```python
from build123d import *

# Parameters (mm, degrees)
F1_DEPTH = 82.55
F2_W     = 25.4
F2_H     = 69.85
F3_DEPTH = 82.55
F4_R     = 20.6375
F4_R_2   = 21.729164
F5_DEPTH = 25.4
F7_DEPTH = 25.4
F8_R     = 23.8125
F9_DEPTH = 25.4


with BuildPart() as f1:
    # F0 (on Front) → F1 (new body)
    with BuildSketch(Plane.XZ):
        Polygon((0, 57.15), (0, 0), (190.5, 0), (190.5, 12.7), (25.4, 12.7), (25.4, 57.15), align=None)
    extrude(amount=F1_DEPTH)

    # F2 (on face) → F3 (join)
    with BuildSketch(Plane.XZ.offset(82.55)):
        with Locations((12.7, 92.075)):
            Rectangle(F2_W, F2_H)
    extrude(amount=-F3_DEPTH)

    # F4 (on face) → F5 (cut)
    with BuildSketch(Plane.XY.offset(12.7)):
        with Locations((76.2, -41.275)):
            Circle(F4_R)
        with Locations((152.4, -41.275)):
            Circle(F4_R_2)
    extrude(amount=-F5_DEPTH, mode=Mode.SUBTRACT)

    # F6 (on face) → F7 (cut)
    with BuildSketch(Plane.YZ.offset(25.4)):
        with BuildLine():
            ThreePointArc((-82.55, 69.85), (-41.275, 111.125), (0, 69.85))
            Line((0, 69.85), (0, 127))
            Line((0, 127), (-82.55, 127))
            Line((-82.55, 127), (-82.55, 69.85))
        make_face()
    extrude(amount=-F7_DEPTH, mode=Mode.SUBTRACT)

    # F8 (on face) → F9 (cut)
    with BuildSketch(Plane.YZ.offset(25.4)):
        with Locations((-41.145787, 70.089974)):
            Circle(F8_R)
    extrude(amount=-F9_DEPTH, mode=Mode.SUBTRACT)


solid = f1.part
```
Geometry check sheet. Reference: the model listing, model coordinates, mm. A direction names the side the tool comes from. Give positions to 0.01 mm unless a question says otherwise; leave off trailing zeros. Order: outer loops, then holes, each group sorted by start corner. A loop starts at its lowest first (then second) coordinate and runs counter-clockwise, first axis right, second up. Notation, with made-up numbers: (-37, 61) - (20, 61) arc R27 ccw to (20, 78) - close; hole circle Ø6 at (27, 14.25). An arc over 180 degrees is marked (long way). Answer in a Markdown table with one row per item. Add a question column.
Q1. Cross-section at B-B, the plane y = -24. Enter the section's corners in (x, z), then the cut area to 3 significant figures.
Q2. Gauge pin test, flat ends, axial feed: pin 1 (8 mm diameter, centred on y = -31.5, z = 89.5, fed in from +X); pin 2 (12 mm diameter, centred on x = 52, y = -66.5, fed in from +Z). Record the tip position at first contact, or that the pin passes through.
Q3. Tool access check on faces 1 (the cylindrical face through (149.57, -19.73, 6.44)), 2 (the flat face through (109, -41, 12.7)). Record the directions out of +Z, -Z, +X, -X, +Y, -Y that give a thin tool (end or side, any length) a straight path to the whole face; none if there is none.
Q4. Cross-section at C-C, the plane z = 73.5. Enter the section's corners in (x, y).
Q5. Material ranges on probe 1 along Y at (x, z) = (76.2, 3.25); probe 2 along X at (y, z) = (-55, 8); probe 3 along Z at (x, y) = (116, -42), recorded low to high. Write a range as from..to.
Q6. Mould release check, pull along Y, two halves, no side actions. Record for faces 3 (the cylindrical face through (12.878, -42.183, 111.115)), 4 (the flat face through (190.5, -41, 6)), 5 (the cylindrical face through (95.884, -35.076, 6.439)), 6 (the flat face through (60, 0, 12)): pulls with the +Y half, pulls with the -Y half, needs draft (parallel to the pull), parting line crosses it, or undercut.
Q7. Cross-section at A-A, the plane x = 76.2. Enter the section's corners in (y, z), then the cut area to 3 significant figures.
Check values:
| question | item | result |
|---|---|---|
| 1 | outline | (0, 0) - (64.91, 0) - (64.91, 12.7) - (25.4, 12.7) - (25.4, 53.57) - (0, 53.57) - close; (0, 86.61) - (25.4, 86.61) - (25.4, 107.34) - (0, 107.34) - close; (87.49, 0) - (139.22, 0) - (139.22, 12.7) - (87.49, 12.7) - close; (165.58, 0) - (190.5, 0) - (190.5, 12.7) - (165.58, 12.7) - close |
| 1 | area | 3,360 mm^2 |
| 2 | pin 1 | stops at x = 25.4 |
| 2 | pin 2 | stops at z = 12.7 |
| 3 | face 1 | +Z, -Z |
| 3 | face 2 | +Z, +X, +Y, -Y |
| 4 | outline | (0, -82.39) - (25.4, -82.39) - (25.4, -64.71) - (0, -64.71) - close; (0, -17.58) - (25.4, -17.58) - (25.4, -0.16) - (0, -0.16) - close |
| 5 | probe 1 | y = -82.55..-61.91, -20.64..0 |
| 5 | probe 2 | x = 0..60.79, 91.61..135.55, 169.25..190.5 |
| 5 | probe 3 | z = 0..12.7 |
| 6 | face 3 | parting line crosses it |
| 6 | face 4 | needs draft |
| 6 | face 5 | undercut |
| 6 | face 6 | pulls with the +Y half |
| 7 | outline | (-82.55, 0) - (-61.91, 0) - (-61.91, 12.7) - (-82.55, 12.7) - close; (-20.64, 0) - (0, 0) - (0, 12.7) - (-20.64, 12.7) - close |
| 7 | area | 524 mm^2 |
